Geometry: final body of the model. Coordinates: model frame, mm. Face numbers are marked on the shaded views. A direction names the side the tool comes from. Coordinates: 2 decimals unless noted, no trailing zeros. Loops run counter-clockwise (first coordinate to the right, second up) from the corner with the lowest first, then second, coordinate; pieces in that order, holes last. Notation, with made-up numbers: (71, -3) - (112, -3) arc R17 cw to (112, 27) - close; hole circle Ø4 at (-21, -31.75). An arc over 180 degrees is marked (long way). Put each result on its own line as item: value. Start each with the question number.
1) Section C-C on y = 0. Output: boundary loops of the cut face in (x, z).
2) Section B-B on z = 30. Output: boundary loops of the cut face in (x, y).
3) Material intervals for line 1 along Y through (x, z) = (-45.5, 5); line 2 along X through (y, z) = (21.5, 28); line 3 along X through (y, z) = (2, 47.5), sorted ascending. Write a range as from..to.
4) Section A-A on x = 0. Output: boundary loops of the cut face in (y, z).
5) Draft query along X for the marked faces 5, 6 and 7. Return one class per face: +X half, -X half, draft (parallel to the pull), parting line (faces both ways), or undercut.
6) Section D-D on z = 22.5. Count the separate pieces of the cut face and the enclosed holes in it, and give its area (3 significant figures).
7) Contact query for a flat-ended pin moving along its axis: pin 1 Ø9 at (x, y) = (17.21, -17.21) entering from -Z. Output: stop coordinate, or through.
8) Reachability of the marked faces 1, 2, 3 and 4 from +Z, -Z, +X, -X, +Y, -Y: full face, straight path, thin tool, end or side. Return the list, or none.
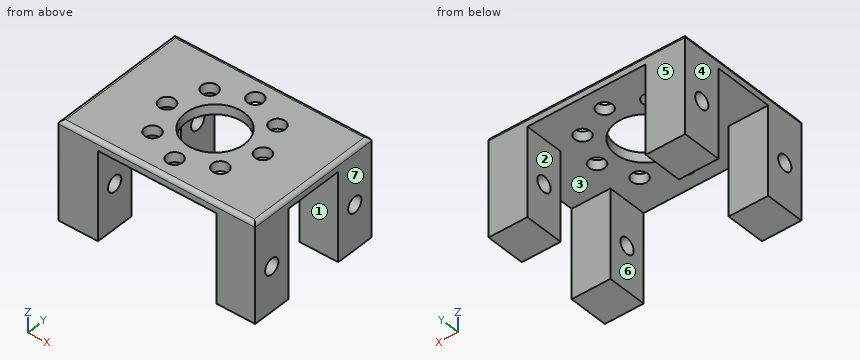
```python
from build123d import *

# Parameters (mm, degrees)
ESBO_O1_W                  = 99.678448554
ESBO_O1_H                  = 70.090169096
ESBO_O1_R                  = 15
ESBO_O1_R_2                = 4
RESSALTO_EXTRUS_O1_DEPTH   = 50
CORTE_EXTRUS_O1_DEPTH      = 79.816915872
CORTE_EXTRUS_O1_DEPTH_BACK = 79.816915872
ESBO_O2_W                  = 60
ESBO_O2_H                  = 45
CORTE_EXTRUS_O2_DEPTH      = 79.816915872
CORTE_EXTRUS_O2_DEPTH_BACK = 79.816915872
CORTE_EXTRUS_O4_DEPTH      = 79.816915872
CORTE_EXTRUS_O4_DEPTH_BACK = 79.816915872
ESBO_O4_R                  = 4
FILETE4_R                  = 2


with BuildPart() as part:
    # Esboço1 → Ressalto-extrusão1 (new body)
    with BuildSketch(Plane.XY):
        Rectangle(ESBO_O1_W, ESBO_O1_H)
        Circle(ESBO_O1_R, mode=Mode.SUBTRACT)
        with Locations((24.33507008, 0)):
            Circle(ESBO_O1_R_2, mode=Mode.SUBTRACT)
        with Locations((17.207493074, -17.207493074)):
            Circle(ESBO_O1_R_2, mode=Mode.SUBTRACT)
        with Locations((0, -24.33507008)):
            Circle(ESBO_O1_R_2, mode=Mode.SUBTRACT)
        with Locations((-17.207493074, -17.207493074)):
            Circle(ESBO_O1_R_2, mode=Mode.SUBTRACT)
        with Locations((-24.33507008, 0)):
            Circle(ESBO_O1_R_2, mode=Mode.SUBTRACT)
        with Locations((-17.207493074, 17.207493074)):
            Circle(ESBO_O1_R_2, mode=Mode.SUBTRACT)
        with Locations((0, 24.33507008)):
            Circle(ESBO_O1_R_2, mode=Mode.SUBTRACT)
        with Locations((17.207493074, 17.207493074)):
            Circle(ESBO_O1_R_2, mode=Mode.SUBTRACT)
    extrude(amount=RESSALTO_EXTRUS_O1_DEPTH)

    # Esboço2 → Corte-extrusão1 (cut, two sides: drawn at the far end of the back side and taken through both)
    with BuildSketch(Plane(origin=(0, 0, 0), x_dir=(1, 0, 0), z_dir=(0, 1, 0)).offset(-CORTE_EXTRUS_O1_DEPTH_BACK)):
        with Locations((0.160775723, -22.5)):
            Rectangle(ESBO_O2_W, ESBO_O2_H)
    extrude(amount=CORTE_EXTRUS_O1_DEPTH + CORTE_EXTRUS_O1_DEPTH_BACK, mode=Mode.SUBTRACT)

    # Esboço3 → Corte-extrusão2 (cut, two sides: drawn at the far end of the back side and taken through both)
    with BuildSketch(Plane(origin=(0, 0, 0), x_dir=(0, 0, -1), z_dir=(1, 0, 0)).offset(-CORTE_EXTRUS_O2_DEPTH_BACK)):
        Polygon((0, 0), (0, 15), (-45, 15), (-45, -15), (0, -15), align=None)
    extrude(amount=CORTE_EXTRUS_O2_DEPTH + CORTE_EXTRUS_O2_DEPTH_BACK, mode=Mode.SUBTRACT)

    # Esboço4 → Corte-extrusão4 (cut, two sides: drawn at the far end of the back side and taken through both)
    with BuildSketch(Plane(origin=(0, 0, 0), x_dir=(0, 0, -1), z_dir=(1, 0, 0)).offset(-CORTE_EXTRUS_O4_DEPTH_BACK)):
        with Locations((-22.5, -25.022542274)):
            Circle(ESBO_O4_R)
        with Locations(Location((-22.5, 25.022542274, 0), (0, 0, 180))):
            Circle(ESBO_O4_R)
    extrude(amount=CORTE_EXTRUS_O4_DEPTH + CORTE_EXTRUS_O4_DEPTH_BACK, mode=Mode.SUBTRACT)

    # Filete4
    filete4_edges = [part.edges().sort_by_distance(p)[0] for p in [
        (-49.839224277, 0, 50),
        (0, -35.045084548, 50),
        (49.839224277, 0, 50),
        (0, 35.045084548, 50),
    ]]
    fillet(filete4_edges, radius=FILETE4_R)


solid = part.part
```
Answer block:
1. outline: (-49.84, 45) - (-28.34, 45) - (-28.34, 50) - (-47.84, 50) arc R2 ccw to (-49.84, 48) - close; (-20.34, 45) - (-15, 45) - (-15, 50) - (-20.34, 50) - close; (15, 45) - (20.34, 45) - (20.34, 50) - (15, 50) - close; (28.34, 45) - (49.84, 45) - (49.84, 48) arc R2 ccw to (47.84, 50) - (28.34, 50) - close
2. outline: (-49.84, -35.05) - (-29.84, -35.05) - (-29.84, -15) - (-49.84, -15) - close; (-49.84, 15) - (-29.84, 15) - (-29.84, 35.05) - (-49.84, 35.05) - close; (30.16, -35.05) - (49.84, -35.05) - (49.84, -15) - (30.16, -15) - close; (30.16, 15) - (49.84, 15) - (49.84, 35.05) - (30.16, 35.05) - close
3. line 1: y = -35.05..-15, 15..35.05
3. line 2: x = -49.84..-29.84, 30.16..49.84
3. line 3: x = -49.84..-27.8, -20.87..-14.87, 14.87..20.87, 27.8..49.84
4. outline: (-35.05, 45) - (-28.34, 45) - (-28.34, 50) - (-33.05, 50) arc R2 ccw to (-35.05, 48) - close; (-20.34, 45) - (-15, 45) - (-15, 50) - (-20.34, 50) - close; (15, 45) - (20.34, 45) - (20.34, 50) - (15, 50) - close; (28.34, 45) - (35.05, 45) - (35.05, 48) arc R2 ccw to (33.05, 50) - (28.34, 50) - close
5. face 5: draft
5. face 6: undercut
5. face 7: +X half
6. separate pieces: 8
6. enclosed holes: 0
6. area: 956 mm²
7. pin 1: stops at z = 45
8. face 1: -Z, +X, -X
8. face 2: -Z, +Y, -Y
8. face 3: -Z
8. face 4: +Z, -Z, -X, +Y, -Y
